from build123d import *

# Parameters (mm, degrees)
BASE_DEPTH                                 = 1.5
BATTERY_STRAP_CUT_REACH                    = 45.853
SKETCH3_W                                  = 2.1
SKETCH3_H                                  = 20
BATTERY_STRAP_FILLET_R                     = 1
BATTERY_STRAP_FILLET_OF_BATTERY_STRAP_OT_R = 1
FILLET2_R                                  = 5
HOLE_CUT_REACH                             = 45.853
SKETCH2_R                                  = 1.6
BOLT_HEAD_CHAMBER_SIZE                     = 1.5
SKETCH4_R                                  = 0.75
MILLING_HOLES_DEPTH                        = 10


with BuildPart() as part:
    # Sketch1 → Base (new body)
    with BuildSketch(Plane.XY):
        Polygon((-19.6, 39.2), (19.6, 39.2), (19.6, -27.6), (15.1, -27.6), (15.1, -25.8), (16.3, -25.8), (16.3, -23.8), (-16.3, -23.8), (-16.3, -25.8), (-15.1, -25.8), (-15.1, -27.6), (-19.6, -27.6), align=None)
    extrude(amount=BASE_DEPTH)

    # Sketch3 → Battery strap cut (cut, up to next)
    with BuildSketch(Plane.XY.offset(1.5), mode=Mode.PRIVATE) as battery_strap_cut_sk1:
        with Locations((-18.55, 0)):
            Rectangle(SKETCH3_W, SKETCH3_H)
    battery_strap_cut_tool1 = extrude(battery_strap_cut_sk1.sketch, amount=-BATTERY_STRAP_CUT_REACH, mode=Mode.PRIVATE) & part.part
    battery_strap_cut = battery_strap_cut_tool1.solids().sort_by_distance((-18.55, 0, 1.5))[0]
    add(battery_strap_cut, mode=Mode.SUBTRACT)

    # Battery strap fillet
    battery_strap_fillet_edges = [part.edges().sort_by_distance(p)[0] for p in [
        (-17.5, 10, 0.75),
        (-17.5, -10, 0.75),
    ]]
    fillet(battery_strap_fillet_edges, radius=BATTERY_STRAP_FILLET_R)

    # Battery strap other side: Battery strap cut across plane
    add(battery_strap_cut.mirror(Plane(origin=(0, 0, 0), x_dir=(0, 0, 1), z_dir=(1, 0, 0))), mode=Mode.SUBTRACT)

    # Battery strap fillet of Battery strap ot
    battery_strap_fillet_of_battery_strap_ot_edges = [part.edges().sort_by_distance(p)[0] for p in [
        (17.5, 10, 0.75),
        (17.5, -10, 0.75),
    ]]
    fillet(battery_strap_fillet_of_battery_strap_ot_edges, radius=BATTERY_STRAP_FILLET_OF_BATTERY_STRAP_OT_R)

    # Fillet2
    fillet2_edges = [part.edges().sort_by_distance(p)[0] for p in [
        (-19.6, 39.2, 0.75),
        (19.6, 39.2, 0.75),
    ]]
    fillet(fillet2_edges, radius=FILLET2_R)

    # Sketch2 → Hole cut (cut, up to next)
    with BuildSketch(Plane.XY.offset(1.5), mode=Mode.PRIVATE) as hole_cut_sk1:
        with Locations((-15.25, 15.25)):
            Circle(SKETCH2_R)
    hole_cut_tool1 = extrude(hole_cut_sk1.sketch, amount=-HOLE_CUT_REACH, mode=Mode.PRIVATE) & part.part
    # Sketch2 → Hole cut (cut, up to next)
    with BuildSketch(Plane.XY.offset(1.5), mode=Mode.PRIVATE) as hole_cut_sk2:
        with Locations((-15.85, 34.85)):
            Circle(SKETCH2_R)
    hole_cut_tool2 = extrude(hole_cut_sk2.sketch, amount=-HOLE_CUT_REACH, mode=Mode.PRIVATE) & part.part
    # Sketch2 → Hole cut (cut, up to next)
    with BuildSketch(Plane.XY.offset(1.5), mode=Mode.PRIVATE) as hole_cut_sk3:
        with Locations((15.85, 34.85)):
            Circle(SKETCH2_R)
    hole_cut_tool3 = extrude(hole_cut_sk3.sketch, amount=-HOLE_CUT_REACH, mode=Mode.PRIVATE) & part.part
    # Sketch2 → Hole cut (cut, up to next)
    with BuildSketch(Plane.XY.offset(1.5), mode=Mode.PRIVATE) as hole_cut_sk4:
        with Locations((15.25, 15.25)):
            Circle(SKETCH2_R)
    hole_cut_tool4 = extrude(hole_cut_sk4.sketch, amount=-HOLE_CUT_REACH, mode=Mode.PRIVATE) & part.part
    # Sketch2 → Hole cut (cut, up to next)
    with BuildSketch(Plane.XY.offset(1.5), mode=Mode.PRIVATE) as hole_cut_sk5:
        with Locations((15.25, -15.25)):
            Circle(SKETCH2_R)
    hole_cut_tool5 = extrude(hole_cut_sk5.sketch, amount=-HOLE_CUT_REACH, mode=Mode.PRIVATE) & part.part
    # Sketch2 → Hole cut (cut, up to next)
    with BuildSketch(Plane.XY.offset(1.5), mode=Mode.PRIVATE) as hole_cut_sk6:
        with Locations((-15.25, -15.25)):
            Circle(SKETCH2_R)
    hole_cut_tool6 = extrude(hole_cut_sk6.sketch, amount=-HOLE_CUT_REACH, mode=Mode.PRIVATE) & part.part
    add(hole_cut_tool1.solids().sort_by_distance((-15.25, 15.25, 1.5))[0], mode=Mode.SUBTRACT)
    add(hole_cut_tool2.solids().sort_by_distance((-15.85, 34.85, 1.5))[0], mode=Mode.SUBTRACT)
    add(hole_cut_tool3.solids().sort_by_distance((15.85, 34.85, 1.5))[0], mode=Mode.SUBTRACT)
    add(hole_cut_tool4.solids().sort_by_distance((15.25, 15.25, 1.5))[0], mode=Mode.SUBTRACT)
    add(hole_cut_tool5.solids().sort_by_distance((15.25, -15.25, 1.5))[0], mode=Mode.SUBTRACT)
    add(hole_cut_tool6.solids().sort_by_distance((-15.25, -15.25, 1.5))[0], mode=Mode.SUBTRACT)

    # Bolt head chamber
    bolt_head_chamber_edges = [part.edges().sort_by_distance(p)[0] for p in [
        (-16.85, 15.25, 1.5),
        (-17.45, 34.85, 1.5),
        (14.25, 34.85, 1.5),
        (13.65, 15.25, 1.5),
        (13.65, -15.25, 1.5),
        (-16.85, -15.25, 1.5),
    ]]
    chamfer(bolt_head_chamber_edges, length=BOLT_HEAD_CHAMBER_SIZE - 0.0001)  # a hair under: the kernel refuses the full size

    # Sketch4 → Milling holes (cut)
    with BuildSketch(Plane.XY.offset(1.5)):
        with Locations((-15.769669914, -24.330330086)):
            Circle(SKETCH4_R)
        with Locations((-15.769669914, -25.269669914)):
            Circle(SKETCH4_R)
        with Locations((15.769669914, -25.269669914)):
            Circle(SKETCH4_R)
        with Locations((15.769669914, -24.330330086)):
            Circle(SKETCH4_R)
    extrude(amount=-MILLING_HOLES_DEPTH, mode=Mode.SUBTRACT)


solid = part.part
Geometry check sheet. Reference: the model listing, model coordinates, mm. A direction names the side the tool comes from. Round coordinates to 2 decimals unless told otherwise and drop trailing zeros. Loops run counter-clockwise (first coordinate to the right, second up) from the corner with the lowest first, then second, coordinate; pieces in that order, holes last.
Item 1: Cross-section at C-C on x = 3.5. Record the boundary of the cut face in (y, z), then the cut area to 3 significant figures.
Item 2: Mould release check, pull along X, two halves, no side actions. Record for faces 3 (the flat face through (19.6, -19, 1)), 4 (the cylindrical face through (16.3, -23.8, 0.8)), 5 (the cylindrical face through (-18.1, 37.77, 0.76)): pulls with the +X half, pulls with the -X half, needs draft (parallel to the pull), parting line crosses it, or undercut.
Item 3: Cross-section at A-A on y = 15.25. Count the separate pieces of the cut face and the enclosed holes in it, then the cut area to 3 significant figures.
Item 4: Gauge pin test, flat end, axial feed: pin 1 (5 mm diameter, centred on x = -15.25, y = -15.25, fed in from +Z). Record the tip position at first contact, or that the pin passes through.
Item 5: Access from +Z, -Z, +X, -X, +Y, -Y to the whole of each face (thin tool, end or side, straight path). Record for faces 1 (the flat face through (15.1, -27, 1)), 2 (the flat face through (0, 39.2, 1)).
Item 6: Thickness scan on line 1 (X direction, y = 14, z = 1.15); line 2 (Y direction, x = 15.25, z = 0.05); line 3 (Y direction, x = 15, z = 1.1). Record the ranges inside material, lowest first.
Answer sheet:
1. outline: (-23.8, 0) - (39.2, 0) - (39.2, 1.5) - (-23.8, 1.5) - close
1. area: 94.5 mm2
2. face 3: pulls with the +X half
2. face 4: undercut
2. face 5: pulls with the -X half
3. separate pieces: 3
3. enclosed holes: 0
3. area: 44.7 mm2
4. pin 1: stops at z = 0.9
5. face 1: +Z, -Z, -Y
5. face 2: +Z, -Z, +X, -X, +Y
6. line 1: x = -19.6 to -17.7, -12.8 to 12.8, 17.7 to 19.6
6. line 2: y = -27.6 to -25.81, -23.79 to -16.9, -13.6 to 13.6, 16.9 to 33.31, 36.39 to 39.16
6. line 3: y = -23.8 to -17.94, -12.56 to 12.56, 17.94 to 32.29, 37.41 to 39.18
